Job drawing, mm, ordinate dimensions from the low corner. One solid piece. A direction names the side the tool comes from. Give positions to 0.01 mm unless a question says otherwise; leave off trailing zeros. Order: outer loops, then holes, each group sorted by start corner. A loop starts at its lowest first (then second) coordinate and runs counter-clockwise, first axis right, second up.
1. Which spindle directions (+Z, -Z, +X, -X, +Y, -Y) get a long thin tool onto all of the face, cutting with end or side? Do the marked faces 1 and 2. Say none if no direction does.
2. Slice it at B-B on y = 20. List the corners of the cut face in (x, z) (1 decimal), and give its area (3 significant figures).
3. Probe line 1 (Y direction, x = 88.9, z = 23.7) (1 decimal); line 2 (Y direction, x = 67, z = 19.5); line 3 (Z direction, x = 74.5, y = 16) (1 decimal). List the from-to ranges inside material, lowest first.
4. Drop a flat-ended pin along its axis: pin 1 Ø8 at (y, z) = (15, 6) entering from -X. Give the stop position or say it passes through.
5. Slice it at A-A on x = 12.7. List the corners of the cut face in (y, z) (1 decimal).
6. Slice it at C-C on z = 23.25. Give the number of separate pieces and of enclosed holes in the cut face, and give its area (3 significant figures).
7. Mould opens along Y. For the marked faces 3, 4, 5 and 6 say: +Y half, -Y half, draft (parallel to the pull), parting line (faces both ways), or undercut.
8. Slice it at D-D on x = 58. List the corners of the cut face in (y, z) (1 decimal).
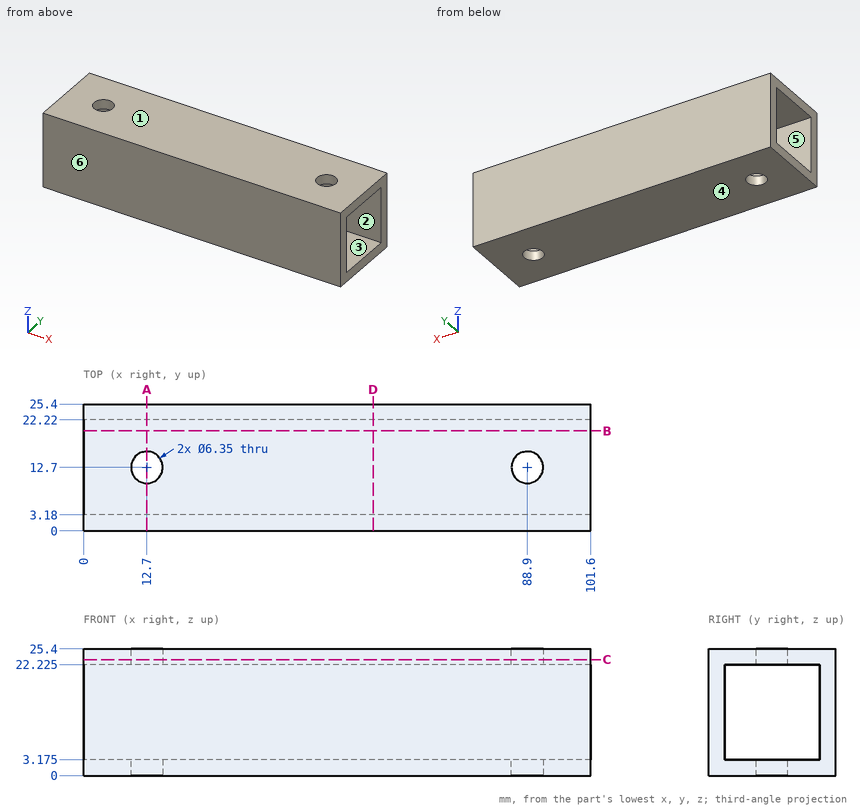
Data:
1. face 1: +Z, +X, -X, +Y, -Y
1. face 2: +X, -X
2. outline: (0, 0) - (101.6, 0) - (101.6, 3.2) - (0, 3.2) - close; (0, 22.2) - (101.6, 22.2) - (101.6, 25.4) - (0, 25.4) - close
2. area: 645 mm2
3. line 1: y = 0 to 9.5, 15.9 to 25.4
3. line 2: y = 0 to 3.18, 22.22 to 25.4
3. line 3: z = 0 to 3.2, 22.2 to 25.4
4. pin 1: stops at x = 0
5. outline: (0, 0) - (9.5, 0) - (9.5, 3.2) - (3.2, 3.2) - (3.2, 22.2) - (9.5, 22.2) - (9.5, 25.4) - (0, 25.4) - close; (15.9, 0) - (25.4, 0) - (25.4, 25.4) - (15.9, 25.4) - (15.9, 22.2) - (22.2, 22.2) - (22.2, 3.2) - (15.9, 3.2) - close
6. separate pieces: 1
6. enclosed holes: 2
6. area: 2,520 mm2
7. face 3: undercut
7. face 4: draft
7. face 5: undercut
7. face 6: -Y half
8. outline: (0, 0) - (25.4, 0) - (25.4, 25.4) - (0, 25.4) - close; hole (3.2, 3.2) - (22.2, 3.2) - (22.2, 22.2) - (3.2, 22.2) - close
